Input: part model. Units: mm. Frame: model coordinates. A direction names the side the tool comes from. Round coordinates to 2 decimals unless told otherwise and drop trailing zeros. Loops run counter-clockwise (first coordinate to the right, second up) from the corner with the lowest first, then second, coordinate; pieces in that order, holes last. Notation, with made-up numbers: (22, -13.5) -> (67, -13.5) arc R29 cw to (67, 19.5) -> close; hole circle Ø11 at (72, 75.5). An arc over 180 degrees is marked (long way). Answer in a Markdown table with one row per item. Add a question column.
Q1. Section D-D, the plane y = -358.5. Output: boundary loops of the cut face in (x, z).
Q2. Section C-C, the plane x = 48. Output: boundary loops of the cut face in (y, z).
Q3. Reachability of faces 1 (the face through (46.321, -503.137, 17.483)), 2 (the face through (0, -504, -64)), 3 (the face through (0, 0, -336)), 4 (the face through (-4.336, 375.489, -315.238)) from +Z, -Z, +X, -X, +Y, -Y: full face, straight path, thin tool, end or side. Return the list, or none.
Q4. Mould query, pull axis Y, two halves, no side actions, for faces 5 (the face through (13.887, -10.648, -481.002)), 6 (the face through (84, -504, 0)), 7 (the face through (0, -553.906, 0)). Classes: pulls with the +Y half, pulls with the -Y half, needs draft (parallel to the pull), parting line crosses it, or undercut.
Q5. Pin query (flat end, axial travel): pin 1 (10 mm diameter, centred on x = 13, z = -233.5, fed in from +Y); pin 2 (10 mm diameter, centred on x = 18, y = 73, fed in from +Z); pin 3 (8 mm diameter, centred on x = 17, y = 244.5, fed in from -Z). Return the tip coordinate at first contact, or that it passes through.
Q6. Section B-B, the plane z = -127.5. Output: boundary loops of the cut face in (x, y), and give its area (3 significant figures).
Q7. Ray query, L1, parallel to Y at x = 0, z = -448; L2, parallel to Y at x = -1, z = -104; L3, parallel to Y at x = -5.5, z = -167.5. Return the intervals inside material, ascending. Write a range as from..to.
Q8. Section A-A, the plane y = 94.5. Output: boundary loops of the cut face in (x, z), and give its area (3 significant figures).
```python
from build123d import *

# Parameters (mm, degrees)
SKETCH2_R           = 20
SKETCH5_R           = 20
BOSS_EXTRUDE1_DEPTH = 553.90605298
SKETCH6_R           = 20
BOSS_EXTRUDE2_DEPTH = 622
SKETCH7_R           = 17.5
CUT_EXTRUDE1_DEPTH  = 286
SKETCH8_R           = 17.5
BOSS_EXTRUDE4_DEPTH = 64
SKETCH11_R          = 17.5
BOSS_EXTRUDE5_DEPTH = 84


with BuildPart() as part:
    # Sweep1: sweep along a path in Sketch3
    with BuildLine(Plane(origin=(0, 0, 0), x_dir=(0, 0, -1), z_dir=(1, 0, 0))) as sweep1_path:
        Line((0, 0), (0, 302.819820908))
        ThreePointArc((0, 302.819820908), (15.565663847, 340.398657675), (53.144500614, 355.964321522))
        Line((53.144500614, 355.964321522), (550.094321522, 355.964321522))
        Line((550.094321522, 355.964321522), (550.094321522, 0.094321522))
    # Sketch2 → Sweep1 (sweep)
    with BuildSketch(Plane(origin=(0, 0, 0), x_dir=(1, 0, 0), z_dir=(0, 1, 0))):
        Circle(SKETCH2_R)
    sweep(path=sweep1_path.line, transition=Transition.RIGHT)

    # Sketch5 → Boss-Extrude1 (add)
    with BuildSketch(Plane.XZ):
        with Locations(Location((0, 0, 0), (0, 0, 90))):
            Circle(SKETCH5_R)
    extrude(amount=BOSS_EXTRUDE1_DEPTH)

    # Sketch6 → Boss-Extrude2 (add)
    with BuildSketch(Plane.XY):
        Circle(SKETCH6_R)
    extrude(amount=-BOSS_EXTRUDE2_DEPTH)

    # Sketch7 → Cut-Extrude1 (cut)
    with BuildSketch(Plane(origin=(0, 0, -622), x_dir=(-1, 0, 0), z_dir=(0, 0, -1))):
        Circle(SKETCH7_R)
    extrude(amount=-CUT_EXTRUDE1_DEPTH, mode=Mode.SUBTRACT)

    # Sketch8 → Boss-Extrude4 (add)
    with BuildSketch(Plane.XY):
        with Locations((0, -503.90605298)):
            Circle(SKETCH8_R)
    extrude(amount=-BOSS_EXTRUDE4_DEPTH)

    # Sketch11 → Boss-Extrude5 (add)
    with BuildSketch(Plane(origin=(0, 0, 0), x_dir=(0, 0, -1), z_dir=(1, 0, 0))):
        with Locations((0, -503.90605298)):
            Circle(SKETCH11_R)
    extrude(amount=BOSS_EXTRUDE5_DEPTH)


solid = part.part
```
Answer block:
| question | item | result |
|---|---|---|
| 1 | outline | circle Ø40 at (0, 0) |
| 2 | outline | circle Ø35 at (-503.91, 0) |
| 3 | face 1 | +X |
| 3 | face 2 | -Z, +X, -X, -Y |
| 3 | face 3 | -Z |
| 3 | face 4 | none |
| 4 | face 5 | undercut |
| 4 | face 6 | needs draft |
| 4 | face 7 | pulls with the -Y half |
| 5 | pin 1 | y = 374.29 |
| 5 | pin 2 | z = 15.2 |
| 5 | pin 3 | z = -565.29 |
| 6 | outline | circle Ø40 at (0, 0); circle Ø40 at (0, 355.96) |
| 6 | area | 2,510 mm^2 |
| 7 | L1 | -20..-17.5, 17.5..20, 335.96..375.96 |
| 7 | L2 | -19.97..19.97, 335.99..375.94 |
| 7 | L3 | -19.23..19.23, 336.74..375.19 |
| 8 | outline | circle Ø40 at (0, -550.09); circle Ø40 at (0, 0) |
| 8 | area | 2,510 mm^2 |
